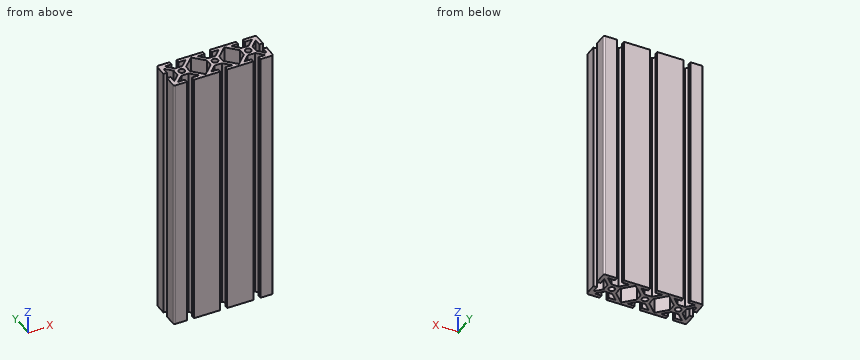
```python
from build123d import *

# Parameters (mm, degrees)
SKETCH1_R      = 3.429
FINALCUT_DEPTH = 301.3074238


with BuildPart() as part:
    # Sketch1 → FinalCut (new body)
    with BuildSketch(Plane.XY):
        with BuildLine():
            Line((-34.036, -19.05), (-34.036, -14.8844))
            Line((-34.036, -14.8844), (-26.089281959, -14.8844))
            Line((-26.089281959, -14.8844), (-33.861681959, -7.112))
            Line((-33.861681959, -7.112), (-42.338318041, -7.112))
            Line((-42.338318041, -7.112), (-50.110718041, -14.8844))
            Line((-50.110718041, -14.8844), (-42.164, -14.8844))
            Line((-42.164, -14.8844), (-42.164, -19.05))
            Line((-42.164, -19.05), (-55.118, -19.05))
            ThreePointArc((-55.118, -19.05), (-56.554840979, -18.454840979), (-57.15, -17.018))
            Line((-57.15, -17.018), (-57.15, -4.064))
            Line((-57.15, -4.064), (-52.9844, -4.064))
            Line((-52.9844, -4.064), (-52.9844, -12.010718041))
            Line((-52.9844, -12.010718041), (-45.212, -4.238318041))
            Line((-45.212, -4.238318041), (-45.212, 4.238318041))
            Line((-45.212, 4.238318041), (-52.9844, 12.010718041))
            Line((-52.9844, 12.010718041), (-52.9844, 4.064))
            Line((-52.9844, 4.064), (-57.15, 4.064))
            Line((-57.15, 4.064), (-57.15, 17.018))
            ThreePointArc((-57.15, 17.018), (-56.554840979, 18.454840979), (-55.118, 19.05))
            Line((-55.118, 19.05), (-42.164, 19.05))
            Line((-42.164, 19.05), (-42.164, 14.8844))
            Line((-42.164, 14.8844), (-50.110718041, 14.8844))
            Line((-50.110718041, 14.8844), (-42.338318041, 7.112))
            Line((-42.338318041, 7.112), (-33.861681959, 7.112))
            Line((-33.861681959, 7.112), (-26.089281959, 14.8844))
            Line((-26.089281959, 14.8844), (-34.036, 14.8844))
            Line((-34.036, 14.8844), (-34.036, 19.05))
            Line((-34.036, 19.05), (-4.064, 19.05))
            Line((-4.064, 19.05), (-4.064, 14.8844))
            Line((-4.064, 14.8844), (-12.010718041, 14.8844))
            Line((-12.010718041, 14.8844), (-4.238318041, 7.112))
            Line((-4.238318041, 7.112), (4.238318041, 7.112))
            Line((4.238318041, 7.112), (12.010718041, 14.8844))
            Line((12.010718041, 14.8844), (4.064, 14.8844))
            Line((4.064, 14.8844), (4.064, 19.05))
            Line((4.064, 19.05), (34.036, 19.05))
            Line((34.036, 19.05), (34.036, 14.8844))
            Line((34.036, 14.8844), (26.089281959, 14.8844))
            Line((26.089281959, 14.8844), (33.861681959, 7.112))
            Line((33.861681959, 7.112), (42.338318041, 7.112))
            Line((42.338318041, 7.112), (50.110718041, 14.8844))
            Line((50.110718041, 14.8844), (42.164, 14.8844))
            Line((42.164, 14.8844), (42.164, 19.05))
            Line((42.164, 19.05), (55.118, 19.05))
            ThreePointArc((55.118, 19.05), (56.554840979, 18.454840979), (57.15, 17.018))
            Line((57.15, 17.018), (57.15, 4.064))
            Line((57.15, 4.064), (52.9844, 4.064))
            Line((52.9844, 4.064), (52.9844, 12.010718041))
            Line((52.9844, 12.010718041), (45.212, 4.238318041))
            Line((45.212, 4.238318041), (45.212, -4.238318041))
            Line((45.212, -4.238318041), (52.9844, -12.010718041))
            Line((52.9844, -12.010718041), (52.9844, -4.064))
            Line((52.9844, -4.064), (57.15, -4.064))
            Line((57.15, -4.064), (57.15, -17.018))
            ThreePointArc((57.15, -17.018), (56.554840979, -18.454840979), (55.118, -19.05))
            Line((55.118, -19.05), (42.164, -19.05))
            Line((42.164, -19.05), (42.164, -14.8844))
            Line((42.164, -14.8844), (50.110718041, -14.8844))
            Line((50.110718041, -14.8844), (42.338318041, -7.112))
            Line((42.338318041, -7.112), (33.861681959, -7.112))
            Line((33.861681959, -7.112), (26.089281959, -14.8844))
            Line((26.089281959, -14.8844), (34.036, -14.8844))
            Line((34.036, -14.8844), (34.036, -19.05))
            Line((34.036, -19.05), (4.064, -19.05))
            Line((4.064, -19.05), (4.064, -14.8844))
            Line((4.064, -14.8844), (12.010718041, -14.8844))
            Line((12.010718041, -14.8844), (4.238318041, -7.112))
            Line((4.238318041, -7.112), (-4.238318041, -7.112))
            Line((-4.238318041, -7.112), (-12.010718041, -14.8844))
            Line((-12.010718041, -14.8844), (-4.064, -14.8844))
            Line((-4.064, -14.8844), (-4.064, -19.05))
            Line((-4.064, -19.05), (-34.036, -19.05))
        make_face()
        with Locations(Location((38.1, 0, 0), (0, 0, 180))):
            Circle(SKETCH1_R, mode=Mode.SUBTRACT)
        with Locations((-38.1, 0)):
            Circle(SKETCH1_R, mode=Mode.SUBTRACT)
        Circle(SKETCH1_R, mode=Mode.SUBTRACT)
        Polygon((-7.112, 4.238318041), (-19.05, 16.176318041), (-30.988, 4.238318041), (-30.988, -4.238318041), (-19.05, -16.176318041), (-7.112, -4.238318041), align=None, mode=Mode.SUBTRACT)
        Polygon((7.112, 4.238318041), (7.112, -4.238318041), (19.05, -16.176318041), (30.988, -4.238318041), (30.988, 4.238318041), (19.05, 16.176318041), align=None, mode=Mode.SUBTRACT)
    extrude(amount=-FINALCUT_DEPTH)


solid = part.part
```
Part model, mm, in its own coordinate system. Round coordinates to 2 decimals unless told otherwise and drop trailing zeros. Loops run counter-clockwise (first coordinate to the right, second up) from the corner with the lowest first, then second, coordinate; pieces in that order, holes last.
Item 1: Drop flat-ended pins along their axis: P1, Ø1, axis at x = -41.5, z = -205.5, coming from the -Y side; P2, Ø1.2, axis at x = 56, z = -168.5, coming from the +Y side; P3, Ø2.5, axis at x = -37.5, z = -107.5, coming from the +Y side. Give the stop position or say it passes through.
Item 2: Cut at B-B, the plane x = 38.1. Give the cut face in (y, z).
Item 3: Cut at C-C, the plane z = -130.5. State how many separate pieces and enclosed holes the cut face has, then the cut area to 3 significant figures.
Item 4: Cut at A-A, the plane y = 0. Give the cut face in (x, z).
Item 5: Drill centre lines: line 1 (X direction, y = -4, z = -201); line 2 (X direction, y = 17, z = -208); line 3 (X direction, y = 0.5, z = -20.5). Where is each one in solid material? Low to high.
A:
1. P1: stops at y = -7.11
1. P2: stops at y = 19.03
1. P3: stops at y = 7.11
2. outline: (-7.11, -301.31) - (-3.43, -301.31) - (-3.43, 0) - (-7.11, 0) - close; (3.43, -301.31) - (7.11, -301.31) - (7.11, 0) - (3.43, 0) - close
3. separate pieces: 1
3. enclosed holes: 5
3. area: 1,980 mm2
4. outline: (-45.21, -301.31) - (-41.53, -301.31) - (-41.53, 0) - (-45.21, 0) - close; (-34.67, -301.31) - (-30.99, -301.31) - (-30.99, 0) - (-34.67, 0) - close; (-7.11, -301.31) - (-3.43, -301.31) - (-3.43, 0) - (-7.11, 0) - close; (3.43, -301.31) - (7.11, -301.31) - (7.11, 0) - (3.43, 0) - close; (30.99, -301.31) - (34.67, -301.31) - (34.67, 0) - (30.99, 0) - close; (41.53, -301.31) - (45.21, -301.31) - (45.21, 0) - (41.53, 0) - close
5. line 1: x = -45.21 to -30.99, -7.11 to 7.11, 30.99 to 45.21
5. line 2: x = -57.15 to -42.16, -34.04 to -4.06, 4.06 to 34.04, 42.16 to 57.15
5. line 3: x = -45.21 to -41.49, -34.71 to -30.99, -7.11 to -3.39, 3.39 to 7.11, 30.99 to 34.71, 41.49 to 45.21
